Input: part model. Units: mm. Frame: model coordinates. A direction names the side the tool comes from. Give positions to 0.01 mm unless a question says otherwise; leave off trailing zeros. Order: outer loops, then holes, each group sorted by start corner. A loop starts at its lowest first (then second) coordinate and runs counter-clockwise, first axis right, second up. Notation, with made-up numbers: (33, -1.5) - (60, -1.5) arc R21 ccw to (60, 10.5) - close; hole circle Ø2 at (64.5, -21). An arc over 180 degrees is marked (long way). Use a Markdown table: item, result.
from build123d import *

# Parameters (mm, degrees)
F0_W     = 63
F0_H     = 52
F1_DEPTH = 1.6
F2_W     = 18.5
F2_H     = 12
F3_DEPTH = 3.5
F4_W     = 10.5
F4_H     = 12
F5_DEPTH = 1
F6_SIZE  = 4


with BuildPart() as f1:
    # F0 (on Top) → F1 (new body)
    with BuildSketch(Plane.XY):
        with Locations((-31.5, 26)):
            Rectangle(F0_W, F0_H)
    extrude(amount=F1_DEPTH)

    # F2 (on face) → F3 (join)
    with BuildSketch(Plane.XY.offset(1.6)):
        with Locations((1.25, 30)):
            Rectangle(F2_W, F2_H)
    extrude(amount=F3_DEPTH)

    # F4 (on face) → F5 (join)
    with BuildSketch(Plane(origin=(0, 0, 1.6), x_dir=(1, 0, 0), z_dir=(0, 0, -1))):
        with Locations((5.25, -30)):
            Rectangle(F4_W, F4_H)
    extrude(amount=F5_DEPTH)

    # F6
    f6_edges = [f1.edges().sort_by_distance(p)[0] for p in [
        (-63, 52, 0.8),
        (0, 52, 0.8),
        (-63, 0, 0.8),
        (0, 0, 0.8),
    ]]
    chamfer(f6_edges, length=F6_SIZE)


solid = f1.part
1. Section query B-B (x = -10). Return loops of the section in (y, z), then the cut area to 3 significant figures.
Response:
| item | result |
|---|---|
| outline | (0, 0) - (52, 0) - (52, 1.6) - (0, 1.6) - close |
| area | 83.2 mm^2 |
2. Set-up query: faces 1 (the face through (5, 30, 0.6)), 2 (the face through (1, 36, 3)), 3 (the face through (-8, 30, 3)). Return all of +Z, -Z, +X, -X, +Y, -Y with unobstructed straight access to the full face (end or side cutting, diameter ignored); none if empty.
Response:
| item | result |
|---|---|
| face 1 | -Z, +X, +Y, -Y |
| face 2 | +Z, +X, +Y |
| face 3 | +Z, -X, +Y, -Y |
3. Section query C-C (z = 3). Return loops of the section in (x, y), then the cut area to 3 significant figures.
Response:
| item | result |
|---|---|
| outline | (-8, 24) - (10.5, 24) - (10.5, 36) - (-8, 36) - close |
| area | 222 mm^2 |
4. Pin query (flat end, axial travel): pin 1 (12 mm diameter, centred on x = -6.5, y = 10, fed in from -Z); pin 2 (5 mm diameter, centred on x = 3, y = 33, fed in from -Z); pin 3 (2 mm diameter, centred on x = 2, z = 2, fed in from +Y); pin 4 (3 mm diameter, centred on y = 32, z = 4, fed in from -X). Return the tip coordinate at first contact, or that it passes through.
Response:
| item | result |
|---|---|
| pin 1 | stops at z = 0 |
| pin 2 | stops at z = 0.6 |
| pin 3 | stops at y = 36 |
| pin 4 | stops at x = -8 |
5. Material intervals for line 1 along X through (y, z) = (34, 4.05); line 2 along X through (y, z) = (44, 0.7); line 3 along Z through (x, y) = (-12.5, 42.5), sorted ascending.
Response:
| item | result |
|---|---|
| line 1 | x = -8 to 10.5 |
| line 2 | x = -63 to 0 |
| line 3 | z = 0 to 1.6 |
6. Section query A-A (y = 33). Return loops of the section in (x, z), then the cut area to 3 significant figures.
Response:
| item | result |
|---|---|
| outline | (-63, 0) - (0, 0) - (0, 0.6) - (10.5, 0.6) - (10.5, 5.1) - (-8, 5.1) - (-8, 1.6) - (-63, 1.6) - close |
| area | 176 mm^2 |
